Input: part model. Units: mm. Frame: model coordinates. Face numbers are marked on the shaded views. Round coordinates to 2 decimals unless told otherwise and drop trailing zeros. Order: outer loops, then holes, each group sorted by start corner. A loop starts at its lowest first (then second) coordinate and runs counter-clockwise, first axis right, second up.
Item 1: Cut plane C-C on x = 36.5. Output: boundary loops of the cut face in (y, z), then the cut area to 3 significant figures.
Item 2: Mould query, pull axis X, two halves, no side actions, for the marked faces 1, 2 and 3. Classes: released by +X, released by -X, zero draft, split by the parting line, or undercut.
Item 3: Cut plane A-A on z = -19. Output: boundary loops of the cut face in (x, y), then the cut area to 3 significant figures.
Item 4: Line query: L1, parallel to X at y = 13.75, z = -20.5; L2, parallel to Z at x = 20.5, y = 3.5; L3, parallel to Z at x = 19, y = 1.5. Output: solid intervals per line, ascending.
Item 5: Cut plane B-B on y = 3.75. Output: boundary loops of the cut face in (x, z), then the cut area to 3 significant figures.
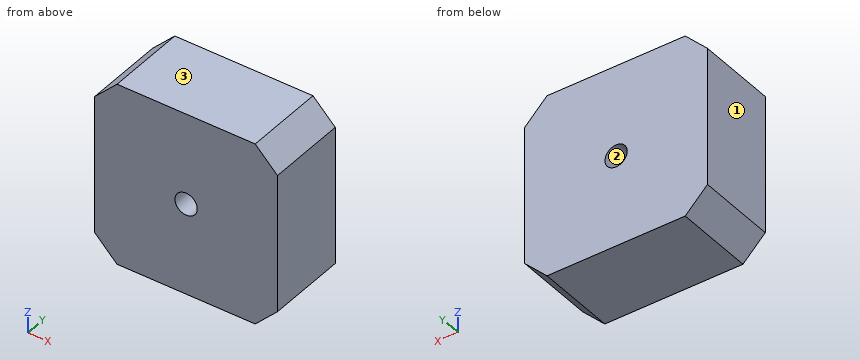
```python
from build123d import *

# Parameters (mm, degrees)
SKETCH1_R           = 2.5
BOSS_EXTRUDE1_DEPTH = 28
SKETCH2_W           = 46.067929507
SKETCH2_H           = 54.310700194
CUT_EXTRUDE1_DEPTH  = 10


with BuildPart() as part:
    # Sketch1 → Boss-Extrude1 (new body)
    with BuildSketch(Plane(origin=(0, 0, 0), x_dir=(1, 0, 0), z_dir=(0, 1, 0))):
        Polygon((5, 0), (36, 0), (41, 5), (41, 36), (36, 41), (5, 41), (0, 36), (0, 5), align=None)
        with Locations(Location((20.5, 20.5, 0), (0, 0, 270))):
            Circle(SKETCH1_R, mode=Mode.SUBTRACT)
    extrude(amount=BOSS_EXTRUDE1_DEPTH)

    # Sketch2 → Cut-Extrude1 (cut)
    with BuildSketch(Plane(origin=(0, 28, 0), x_dir=(1, 0, 0), z_dir=(0, 1, 0))):
        with Locations((20.912138535, 21.370070239)):
            Rectangle(SKETCH2_W, SKETCH2_H)
    extrude(amount=-CUT_EXTRUDE1_DEPTH, mode=Mode.SUBTRACT)


solid = part.part
```
From the geometry:
1. outline: (0, -40.5) - (18, -40.5) - (18, -0.5) - (0, -0.5) - close
1. area: 720 mm2
2. face 1: released by -X
2. face 2: undercut
2. face 3: zero draft
3. outline: (0, 0) - (18.5, 0) - (18.5, 18) - (0, 18) - close; (22.5, 0) - (41, 0) - (41, 18) - (22.5, 18) - close
3. area: 666 mm2
4. L1: x = 0 to 18, 23 to 41
4. L2: z = -41 to -23, -18 to 0
4. L3: z = -41 to -22.5, -18.5 to 0
5. outline: (0, -36) - (5, -41) - (36, -41) - (41, -36) - (41, -5) - (36, 0) - (5, 0) - (0, -5) - close; hole circle Ø5 at (20.5, -20.5)
5. area: 1,610 mm2
